```python
from build123d import *

# Parameters (mm, degrees)
SKETCH1_W           = 22
SKETCH1_H           = 28
SKETCH1_R           = 1.5
SKETCH1_R_2         = 0.55
BOSS_EXTRUDE1_DEPTH = 1.8
SKETCH2_W           = 5.3
SKETCH2_H           = 4.5
BOSS_EXTRUDE2_DEPTH = 1
CHAMFER1_SIZE       = 0.5
CHAMFER2_SIZE       = 0.1
SKETCH3_R           = 0.375
CUT_EXTRUDE1_DEPTH  = 0.1


with BuildPart() as part:
    # Sketch1 → Boss-Extrude1 (new body)
    with BuildSketch(Plane(origin=(0, 0, 0), x_dir=(1, 0, 0), z_dir=(0, 1, 0))):
        Rectangle(SKETCH1_W, SKETCH1_H)
        with Locations(Location((-9, 12, 0), (0, 0, 270))):
            Circle(SKETCH1_R, mode=Mode.SUBTRACT)
        with Locations(Location((9, 12, 0), (0, 0, 270))):
            Circle(SKETCH1_R, mode=Mode.SUBTRACT)
        with Locations(Location((9, 1, 0), (0, 0, 270))):
            Circle(SKETCH1_R, mode=Mode.SUBTRACT)
        with Locations(Location((-9, 1, 0), (0, 0, 270))):
            Circle(SKETCH1_R, mode=Mode.SUBTRACT)
        with Locations(Location((-8.89, -12.5, 0), (0, 0, 270))):
            Circle(SKETCH1_R_2, mode=Mode.SUBTRACT)
        with Locations(Location((-6.35, -12.5, 0), (0, 0, 270))):
            Circle(SKETCH1_R_2, mode=Mode.SUBTRACT)
        with Locations(Location((-3.81, -12.5, 0), (0, 0, 270))):
            Circle(SKETCH1_R_2, mode=Mode.SUBTRACT)
        with Locations(Location((-1.27, -12.5, 0), (0, 0, 270))):
            Circle(SKETCH1_R_2, mode=Mode.SUBTRACT)
        with Locations(Location((1.27, -12.5, 0), (0, 0, 270))):
            Circle(SKETCH1_R_2, mode=Mode.SUBTRACT)
        with Locations(Location((3.81, -12.5, 0), (0, 0, 270))):
            Circle(SKETCH1_R_2, mode=Mode.SUBTRACT)
        with Locations(Location((6.35, -12.5, 0), (0, 0, 270))):
            Circle(SKETCH1_R_2, mode=Mode.SUBTRACT)
        with Locations(Location((8.89, -12.5, 0), (0, 0, 270))):
            Circle(SKETCH1_R_2, mode=Mode.SUBTRACT)
    extrude(amount=BOSS_EXTRUDE1_DEPTH)

    # Sketch2 → Boss-Extrude2 (add)
    with BuildSketch(Plane(origin=(0, 1.8, 0), x_dir=(1, 0, 0), z_dir=(0, 1, 0))):
        with Locations((0, 6.5)):
            Rectangle(SKETCH2_W, SKETCH2_H)
    extrude(amount=BOSS_EXTRUDE2_DEPTH)

    # Chamfer1
    chamfer1_edges = [part.edges().sort_by_distance(p)[0] for p in [
        (0, 1.8, -8.75),
        (0, 1.8, -4.25),
    ]]
    chamfer(chamfer1_edges, length=CHAMFER1_SIZE)

    # Chamfer2
    chamfer2_edges = [part.edges().sort_by_distance(p)[0] for p in [
        (2.65, 2.8, -6.5),
        (0, 2.8, -8.75),
        (-2.65, 2.8, -6.5),
        (0, 2.8, -4.25),
    ]]
    chamfer(chamfer2_edges, length=CHAMFER2_SIZE)

    # Sketch3 → Cut-Extrude1 (cut)
    with BuildSketch(Plane(origin=(0, 2.8, 0), x_dir=(1, 0, 0), z_dir=(0, 1, 0))):
        with Locations(Location((1.8, 7.9, 0), (0, 0, 270))):
            Circle(SKETCH3_R)
    extrude(amount=-CUT_EXTRUDE1_DEPTH, mode=Mode.SUBTRACT)


solid = part.part
```
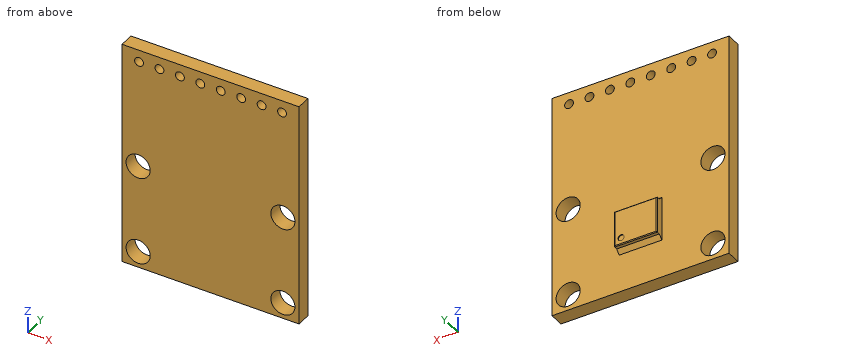
Geometry: final body of the model. Coordinates: model frame, mm. Round coordinates to 2 decimals unless told otherwise and drop trailing zeros. Loops run counter-clockwise (first coordinate to the right, second up) from the corner with the lowest first, then second, coordinate; pieces in that order, holes last. Notation, with made-up numbers: (87.25, 64.5) -> (100.25, 64.5) arc R22 cw to (100.25, 96.5) -> close; hole circle Ø1 at (-14, 15). An arc over 180 degrees is marked (long way). Use one line per item in the form item = value.
Item 1: Cut plane C-C on y = 0.55. Give the number of separate pieces and of enclosed holes in the cut face, then the cut area to 3 significant figures.
Evaluation:
separate_pieces = 1
enclosed_holes = 12
area = 580 mm2
Item 2: Cut plane A-A on z = -1. Output: boundary loops of the cut face in (x, y).
Evaluation:
outline = (-11, 0) -> (-10.5, 0) -> (-10.5, 1.8) -> (-11, 1.8) -> close; (-7.5, 0) -> (7.5, 0) -> (7.5, 1.8) -> (-7.5, 1.8) -> close; (10.5, 0) -> (11, 0) -> (11, 1.8) -> (10.5, 1.8) -> close
Item 3: Cut plane D-D on x = -8. Output: boundary loops of the cut face in (y, z), then the cut area to 3 significant figures.
Evaluation:
outline = (0, -14) -> (1.8, -14) -> (1.8, -13.12) -> (0, -13.12) -> close; (0, -10.88) -> (1.8, -10.88) -> (1.8, -2.12) -> (0, -2.12) -> close; (0, 0.12) -> (1.8, 0.12) -> (1.8, 14) -> (0, 14) -> close
area = 42.4 mm2
Item 4: Cut plane B-B on x = -1.27. Output: boundary loops of the cut face in (y, z), then the cut area to 3 significant figures.
Evaluation:
outline = (0, -14) -> (1.8, -14) -> (1.8, -9.25) -> (2.3, -8.75) -> (2.7, -8.75) -> (2.8, -8.65) -> (2.8, -4.35) -> (2.7, -4.25) -> (2.3, -4.25) -> (1.8, -3.75) -> (1.8, 11.95) -> (0, 11.95) -> close; (0, 13.05) -> (1.8, 13.05) -> (1.8, 14) -> (0, 14) -> close
area = 53.2 mm2
Item 5: Material intervals for probe 1 along Z at (x, y) = (-10, 0.7); probe 2 along Y at (x, z) = (-4.5, 11.75); probe 3 along Z at (x, y) = (-8.5, 0.2), sorted ascending.
Evaluation:
probe_1 = -14 to -13.12, -10.88 to -2.12, 0.12 to 14
probe_2 = 0 to 1.8
probe_3 = -14 to -13.41, -10.59 to -2.41, 0.41 to 12.11, 12.89 to 14
Item 6: Contact query for flat-ended pins moving along their axis: pin 1 Ø0.7 at (y, z) = (2.5, -6.5) entering from -X; pin 2 Ø5 at (x, z) = (-9, -1) entering from -Y; pin 3 Ø0.7 at (x, z) = (-3.81, 12.5) entering from -Y; pin 4 Ø11 at (x, z) = (3, 3) entering from +Y. Output: stop coordinate, or through.
Evaluation:
pin_1 = -2.65
pin_2 = 0
pin_3 = through
pin_4 = 1.8
